Source: CAD feature listing. Evaluate the final solid. Frame: model axes, mm. Coordinates: 2 decimals unless noted, no trailing zeros. Write each loop counter-clockwise with the first axis right and the second up, starting at its lowest first coordinate (ties: lowest second). Pieces come first, ordered by that corner, then holes. Notation, with made-up numbers: (-9, -24) -> (30, -24) arc R35 cw to (30, 10) -> close; hole circle Ø6 at (44.5, -32). An arc over 180 degrees is marked (long way). Write item = value, one per line.
from build123d import *

# Parameters (mm, degrees)
F0_W     = 124.5182976127
F0_H     = 89.5412452519
F1_DEPTH = 45.72
F3_D     = 6.5278
F5_D     = 6.35


with BuildPart() as f1:
    # F0 (on Top) → F1 (new body)
    with BuildSketch(Plane.XY):
        with Locations((8.5693784058, 0.2623293549)):
            Rectangle(F0_W, F0_H)
    extrude(amount=F1_DEPTH)

    # F3 (through all)
    with Locations(Plane.XY.offset(45.72)):
        with Locations((-22.6416923106, -17.2483026981)):
            Hole(F3_D / 2)

    # F5 (through all)
    with Locations(Plane.XY.offset(45.72)):
        with Locations((32.5962975621, -11.8062160909)):
            Hole(F5_D / 2)


solid = f1.part
1) Cut plane A-A, the plane x = -22. Output: boundary loops of the cut face in (y, z).
Answer block:
outline = (-44.51, 0) -> (-20.45, 0) -> (-20.45, 45.72) -> (-44.51, 45.72) -> close; (-14.05, 0) -> (45.03, 0) -> (45.03, 45.72) -> (-14.05, 45.72) -> close
2) Pull-direction query (Y, two-part tool) for faces 1 (the flat face through (8, -44.508, 23)), 2 (the flat face through (8, 1, 45.72)), 3 (the cylindrical face through (35.77, -11.67, 22.54)); classes: +Y half, -Y half, draft (parallel to the pull), parting line (faces both ways), or undercut.
Answer block:
face_1 = -Y half
face_2 = draft
face_3 = undercut
3) Material intervals for probe 1 along X at (y, z) = (-11.5, 39); probe 2 along Y at (x, z) = (31.5, 38), sorted ascending. Write a range as [from, to].
Answer block:
probe_1 = [-53.69, 29.44], [35.76, 70.83]
probe_2 = [-44.51, -14.79], [-8.83, 45.03]
4) First-contact query: pin 1 Ø7.5 at (x, y) = (-22.64, -17.25) entering from -Z. Flat tip, straight axial feed; report the tip coordinate or a pass-through.
Answer block:
pin_1 = 0
